Geometry check sheet. Reference: the model listing, model coordinates, mm. A direction names the side the tool comes from. Coordinates: 2 decimals unless noted, no trailing zeros. Write each loop counter-clockwise with the first axis right and the second up, starting at its lowest first coordinate (ties: lowest second). Pieces come first, ordered by that corner, then holes. Notation, with made-up numbers: M -38,40 L -13,40 A7 ccw -13,48 Z; hole C 62,62.5 d2. An arc over 180 degrees is marked long. Write each question's results on one line, items separated by ' | '.
```python
from build123d import *

# Parameters (mm, degrees)
SKETCH1_W               = 100
SKETCH1_H               = 206
BOSS_EXTRUDE1_DEPTH     = 6
SKETCH2_W               = 6
SKETCH2_H               = 20
CUT_EXTRUDE1_DEPTH      = 10
LPATTERN1_COUNT         = 5
LPATTERN1_PITCH         = 40
MIRROR2_COPY_1_SKETCH_W = 6
MIRROR2_COPY_1_SKETCH_H = 20
MIRROR2_COPY_1_DEPTH    = 10
MIRROR2_COPY_2_SKETCH_W = 6
MIRROR2_COPY_2_SKETCH_H = 20
MIRROR2_COPY_2_DEPTH    = 10
MIRROR2_COPY_3_SKETCH_W = 6
MIRROR2_COPY_3_SKETCH_H = 20
MIRROR2_COPY_3_DEPTH    = 10
MIRROR2_COPY_4_SKETCH_W = 6
MIRROR2_COPY_4_SKETCH_H = 20
MIRROR2_COPY_4_DEPTH    = 10
SKETCH4_W               = 20
SKETCH4_H               = 6
CUT_EXTRUDE2_DEPTH      = 10
LPATTERN2_COUNT         = 3
LPATTERN2_PITCH         = 40


with BuildPart() as part:
    # Sketch1 → Boss-Extrude1 (new body)
    with BuildSketch(Plane.XY):
        with Locations((40, 96.427419355)):
            Rectangle(SKETCH1_W, SKETCH1_H)
    extrude(amount=BOSS_EXTRUDE1_DEPTH)

    # Sketch2 → Cut-Extrude1 (cut)
    with BuildSketch(Plane.XY):
        with Locations((-7, 3.427419355)):
            Rectangle(SKETCH2_W, SKETCH2_H)
    cut_extrude1 = extrude(amount=CUT_EXTRUDE1_DEPTH, mode=Mode.SUBTRACT)

    # LPattern1: Cut-Extrude1 ×5
    with Locations(*[(0, i * LPATTERN1_PITCH, 0) for i in range(1, LPATTERN1_COUNT)]):
        add(cut_extrude1, mode=Mode.SUBTRACT)

    # Mirror2: Cut-Extrude1 across plane
    add(cut_extrude1.mirror(Plane(origin=(40, 0, 0), x_dir=(0, 0, 1), z_dir=(1, 0, 0))), mode=Mode.SUBTRACT)

    # Mirror2 copy 1 sketch → Mirror2 copy 1 (cut)
    with BuildSketch(Plane(origin=(80, 40, 0), x_dir=(-1, 0, 0), z_dir=(0, 0, 1))):
        with Locations((-7, -3.427419355)):
            Rectangle(MIRROR2_COPY_1_SKETCH_W, MIRROR2_COPY_1_SKETCH_H)
    extrude(amount=MIRROR2_COPY_1_DEPTH, mode=Mode.SUBTRACT)

    # Mirror2 copy 2 sketch → Mirror2 copy 2 (cut)
    with BuildSketch(Plane(origin=(80, 80, 0), x_dir=(-1, 0, 0), z_dir=(0, 0, 1))):
        with Locations((-7, -3.427419355)):
            Rectangle(MIRROR2_COPY_2_SKETCH_W, MIRROR2_COPY_2_SKETCH_H)
    extrude(amount=MIRROR2_COPY_2_DEPTH, mode=Mode.SUBTRACT)

    # Mirror2 copy 3 sketch → Mirror2 copy 3 (cut)
    with BuildSketch(Plane(origin=(80, 120, 0), x_dir=(-1, 0, 0), z_dir=(0, 0, 1))):
        with Locations((-7, -3.427419355)):
            Rectangle(MIRROR2_COPY_3_SKETCH_W, MIRROR2_COPY_3_SKETCH_H)
    extrude(amount=MIRROR2_COPY_3_DEPTH, mode=Mode.SUBTRACT)

    # Mirror2 copy 4 sketch → Mirror2 copy 4 (cut)
    with BuildSketch(Plane(origin=(80, 160, 0), x_dir=(-1, 0, 0), z_dir=(0, 0, 1))):
        with Locations((-7, -3.427419355)):
            Rectangle(MIRROR2_COPY_4_SKETCH_W, MIRROR2_COPY_4_SKETCH_H)
    extrude(amount=MIRROR2_COPY_4_DEPTH, mode=Mode.SUBTRACT)

    # Sketch4 → Cut-Extrude2 (cut)
    with BuildSketch(Plane.XY.offset(6)):
        with Locations((0, -3.572580645)):
            Rectangle(SKETCH4_W, SKETCH4_H)
    cut_extrude2 = extrude(amount=-CUT_EXTRUDE2_DEPTH, mode=Mode.SUBTRACT)

    # LPattern2: Cut-Extrude2 ×3
    with Locations(*[(i * LPATTERN2_PITCH, 0, 0) for i in range(1, LPATTERN2_COUNT)]):
        add(cut_extrude2, mode=Mode.SUBTRACT)


solid = part.part
```
Q1. Sectioned sample at B-B on x = 43.5. Record the cut outline in (y, z), and give its area (3 significant figures).
Geometry check:
outline: M -0.57,0 L 199.43,0 L 199.43,6 L -0.57,6 Z | area: 1,200 mm2
Q2. Sectioned sample at A-A on y = 119. Record the cut outline in (x, z), and give its area (3 significant figures).
Geometry check:
outline: M -4,0 L 84,0 L 84,6 L -4,6 Z | area: 528 mm2
Q3. Access from +Z, -Z, +X, -X, +Y, -Y to the whole of each face (thin tool, end or side, straight path). Record for faces 4 (the flat face through (87, 13.427, 3)), 5 (the flat face through (-7, 153.427, 3)), 6 (the flat face through (10, -4, 3)), 7 (the flat face through (87, 53.427, 3)).
Geometry check:
face 4: +Z, -Z, +X, -Y | face 5: +Z, -Z, -X | face 6: +Z, -Z, -X, -Y | face 7: +Z, -Z, +X
Q4. Scan lines: probe 1 along Y at (x, z) = (85.5, 2.9); probe 2 along X at (y, z) = (51.5, 1.1); probe 3 along Y at (x, z) = (46.5, 5.75). Record each from-to range of solid material in increasing order.
Geometry check:
probe 1: y = 13.43 to 33.43, 53.43 to 73.43, 93.43 to 113.43, 133.43 to 153.43, 173.43 to 199.43 | probe 2: x = -4 to 84 | probe 3: y = -0.57 to 199.43
Q5. Depth check by flat-ended pin: P1, Ø1.8, axis at y = -4, z = 4, coming from the +X side; P2, Ø1.8, axis at x = -6.5, z = 3, coming from the -Y side; P3, Ø1.8, axis at y = -5, z = 2.5, coming from the -X side. Enter the tip coordinate at first touch or a pass-through.
Geometry check:
P1: stops at x = 70 | P2: stops at y = 13.43 | P3: stops at x = 10
Q6. Mould release check, pull along X, two halves, no side actions. Record for faces 1 (the flat face through (50, -4, 3)), 2 (the flat face through (84, 6, 3)), 3 (the flat face through (-7, 133.427, 3)): pulls with the +X half, pulls with the -X half, needs draft (parallel to the pull), parting line crosses it, or undercut.
Geometry check:
face 1: undercut | face 2: pulls with the +X half | face 3: needs draft
